from build123d import *

# Parameters (mm, degrees)
SKETCH1_W           = 90
SKETCH1_H           = 90
BOSS_EXTRUDE1_DEPTH = 25
SKETCH2_W           = 50
SKETCH2_H           = 25
BOSS_EXTRUDE2_DEPTH = 90
CUT_EXTRUDE1_DEPTH  = 114
BOSS_EXTRUDE3_DEPTH = 90
CUT_EXTRUDE2_DEPTH  = 90
CUT_EXTRUDE3_DEPTH  = 7
SKETCH12_W          = 60
SKETCH12_H          = 3.762713397
CUT_EXTRUDE4_DEPTH  = 7
SKETCH13_W          = 60
SKETCH13_H          = 6.597800351
BOSS_EXTRUDE4_DEPTH = 4
SKETCH15_W          = 60
SKETCH15_H          = 4.875511562
BOSS_EXTRUDE5_DEPTH = 6
CUT_EXTRUDE5_DEPTH  = 105
CUT_EXTRUDE6_DEPTH  = 105
CUT_EXTRUDE7_DEPTH  = 105
CUT_EXTRUDE8_DEPTH  = 105
SKETCH20_R          = 5.002398859
BOSS_EXTRUDE6_DEPTH = 5
SKETCH21_R          = 5.013240391
BOSS_EXTRUDE7_DEPTH = 5
CUT_EXTRUDE9_DEPTH  = 110
CUT_EXTRUDE10_DEPTH = 110
BOSS_EXTRUDE8_DEPTH = 90


with BuildPart() as part:
    # Sketch1 → Boss-Extrude1 (new body)
    with BuildSketch(Plane(origin=(0, 0, 0), x_dir=(1, 0, 0), z_dir=(0, 1, 0))):
        with Locations((-396.44486692, -394.733840304)):
            Rectangle(SKETCH1_W, SKETCH1_H)
    extrude(amount=BOSS_EXTRUDE1_DEPTH)

    # Sketch2 → Boss-Extrude2 (add)
    with BuildSketch(Plane(origin=(-351.44486692, 0, 0), x_dir=(0, 0, -1), z_dir=(1, 0, 0))):
        with Locations((-324.733840304, 12.5)):
            Rectangle(SKETCH2_W, SKETCH2_H)
    extrude(amount=-BOSS_EXTRUDE2_DEPTH)

    # Sketch3 → Cut-Extrude1 (cut)
    with BuildSketch(Plane(origin=(-351.44486692, 0, 0), x_dir=(0, 0, -1), z_dir=(1, 0, 0))):
        Polygon((-439.733840304, 0), (-431.428630034, 25), (-426.683614644, 23.423665978), (-432.80411144, 5), (-422.80411144, 5), (-417.80411144, 5), (-409.869768155, 28.88363156), (-456.556935105, 33.347834294), align=None)
    extrude(amount=-CUT_EXTRUDE1_DEPTH, mode=Mode.SUBTRACT)

    # Sketch6 → Boss-Extrude3 (add)
    with BuildSketch(Plane(origin=(-351.44486692, 0, 0), x_dir=(0, 0, -1), z_dir=(1, 0, 0))):
        Polygon((-417.80411144, 5), (-402.036905068, 52.448869357), (-397.292018132, 50.872148719), (-412.958326169, 3.726916659), align=None)
    extrude(amount=-BOSS_EXTRUDE3_DEPTH)

    # Sketch8 → Cut-Extrude2 (cut)
    with BuildSketch(Plane.ZY.offset(441.44486692)):
        Polygon((402.036905068, 52.448869357), (417.80411144, 5), (422.667757436, 11.843524049), (408.096373886, 67.204399508), align=None)
    extrude(amount=-CUT_EXTRUDE2_DEPTH, mode=Mode.SUBTRACT)

    # Sketch11 → Cut-Extrude3 (cut)
    with BuildSketch(Plane(origin=(0, 131.563601718, 396.027305256), x_dir=(1, 0, 0), z_dir=(0, 0.31526680439845073, 0.9490030779952134))):
        Polygon((-396.44486692, -112.290048567), (-366.44486692, -112.290048567), (-366.44486692, -132.290048567), (-426.44486692, -132.290048567), (-426.44486692, -112.290048567), align=None)
    extrude(amount=-CUT_EXTRUDE3_DEPTH, mode=Mode.SUBTRACT)

    # Sketch12 → Cut-Extrude4 (cut)
    with BuildSketch(Plane(origin=(0, 131.563601718, 396.027305256), x_dir=(1, 0, 0), z_dir=(0, 0.31526680439845073, 0.9490030779952134))):
        with Locations((-396.44486692, -134.171405266)):
            Rectangle(SKETCH12_W, SKETCH12_H)
    extrude(amount=-CUT_EXTRUDE4_DEPTH, mode=Mode.SUBTRACT)

    # Sketch13 → Boss-Extrude4 (add)
    with BuildSketch(Plane(origin=(0, 5, 0), x_dir=(1, 0, 0), z_dir=(0, 1, 0))):
        with Locations((-396.44486692, -433.995536892)):
            Rectangle(SKETCH13_W, SKETCH13_H)
    extrude(amount=-BOSS_EXTRUDE4_DEPTH)

    # Sketch15 → Boss-Extrude5 (add)
    with BuildSketch(Plane(origin=(0, 131.563601718, 396.027305256), x_dir=(1, 0, 0), z_dir=(0, 0.31526680439845073, 0.9490030779952134))):
        with Locations((-396.44486692, -133.615006183)):
            Rectangle(SKETCH15_W, SKETCH15_H)
    extrude(amount=-BOSS_EXTRUDE5_DEPTH)

    # Sketch16 → Cut-Extrude5 (cut)
    with BuildSketch(Plane.ZY.offset(441.44486692)):
        Polygon((299.733840304, 25), (405.889304299, 25), (320.938870245, 45.924702762), (282.519842095, 35.688976285), (299.733840304, -6.375653077), (299.733840304, 0), (299.733840304, 13.612271354), align=None)
        Polygon((409.673433828, 13.612271354), (405.889304299, 25), (299.733840304, 25), (299.733840304, 13.612271354), align=None)
    extrude(amount=-CUT_EXTRUDE5_DEPTH, mode=Mode.SUBTRACT)

    # Sketch17 → Cut-Extrude6 (cut)
    with BuildSketch(Plane(origin=(-351.44486692, 0, 0), x_dir=(0, 0, -1), z_dir=(1, 0, 0))):
        Polygon((-354.703637066, 13.612271354), (-354.703637066, -9.141758862), (-285.710269568, -9.141758862), (-285.710269568, 26.661614512), (-354.703637066, 26.661614512), align=None)
    extrude(amount=-CUT_EXTRUDE6_DEPTH, mode=Mode.SUBTRACT)

    # Sketch18 → Cut-Extrude7 (cut)
    with BuildSketch(Plane(origin=(0, 125.526947543, 377.753141183), x_dir=(1, 0, 0), z_dir=(0, 0.3153441274409663, 0.9489773871323255))):
        Polygon((-441.44486692, -77.007186028), (-436.44486692, -77.007186028), (-441.44486692, -82.007186028), align=None)
    extrude(amount=-CUT_EXTRUDE7_DEPTH, mode=Mode.SUBTRACT)

    # Sketch19 → Cut-Extrude8 (cut)
    with BuildSketch(Plane(origin=(0, 125.526947543, 377.753141183), x_dir=(1, 0, 0), z_dir=(0, 0.3153441274409663, 0.9489773871323255))):
        Polygon((-351.44486692, -82.007186028), (-351.44486692, -77.007186028), (-356.44486692, -77.007186028), align=None)
    extrude(amount=-CUT_EXTRUDE8_DEPTH, mode=Mode.SUBTRACT)

    # Sketch20 → Boss-Extrude6 (add)
    with BuildSketch(Plane(origin=(0, 125.526947543, 377.753141183), x_dir=(1, 0, 0), z_dir=(0, 0.3153441274409663, 0.9489773871323255))):
        with Locations((-436.44486692, -82.007186028)):
            Circle(SKETCH20_R)
    extrude(amount=-BOSS_EXTRUDE6_DEPTH)

    # Sketch21 → Boss-Extrude7 (add)
    with BuildSketch(Plane(origin=(0, 125.526947543, 377.753141183), x_dir=(1, 0, 0), z_dir=(0, 0.3153441274409663, 0.9489773871323255))):
        with Locations((-356.44486692, -82.007186028)):
            Circle(SKETCH21_R)
    extrude(amount=-BOSS_EXTRUDE7_DEPTH)

    # Sketch22 → Cut-Extrude9 (cut)
    with BuildSketch(Plane.ZY.offset(441.44486692)):
        with BuildLine():
            Line((352.286663655, 0), (351.925563617, 18.995212977))
            Line((351.925563617, 18.995212977), (405.563075233, 20.014865007))
            Line((405.563075233, 20.014865007), (409.673433828, 13.612271354))
            add(Edge.make_bspline(
                [(409.673433828, 13.612271354), (391.693864934, -0.348112278), (371.968229932, 0.006592141), (352.286663655, 0)],
                knots=[0, 0, 0, 0, 1, 1, 1, 1], degree=3))
        make_face()
    extrude(amount=-CUT_EXTRUDE9_DEPTH, mode=Mode.SUBTRACT)

    # Sketch23 → Cut-Extrude10 (cut)
    with BuildSketch(Plane(origin=(-351.44486692, 0, 0), x_dir=(0, 0, -1), z_dir=(1, 0, 0))):
        Polygon((-432.207797356, 6.794999958), (-432.80411144, 5), (-433.434645049, 3.101993844), (-418.434799695, 3.102045226), (-417.80411144, 5), (-417.309872164, 6.487333538), align=None)
    extrude(amount=-CUT_EXTRUDE10_DEPTH, mode=Mode.SUBTRACT)

    # Sketch24 → Boss-Extrude8 (add)
    with BuildSketch(Plane(origin=(-351.44486692, 0, 0), x_dir=(0, 0, -1), z_dir=(1, 0, 0))):
        Polygon((-439.733840304, 0), (-440.364373913, -1.898006156), (-355.334170675, -1.898006156), (-354.703637066, 0), align=None)
    extrude(amount=-BOSS_EXTRUDE8_DEPTH)


solid = part.part
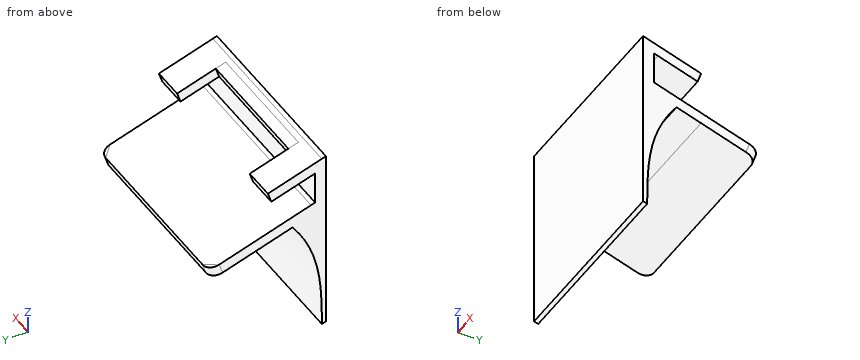
Geometry check sheet. Reference: the model listing, model coordinates, mm. Give positions to 0.01 mm unless a question says otherwise; leave off trailing zeros. Loops run counter-clockwise (first coordinate to the right, second up) from the corner with the lowest first, then second, coordinate; pieces in that order, holes last.
(1) Thickness scan on L1, parallel to X at y = 17, z = 434; L2, parallel to X at y = 1.5, z = 428; L3, parallel to Y at x = -361, z = 424.5. Record the ranges inside material, lowest first.
From the geometry:
L1: x = -441.44 to -426.44, -366.44 to -351.44
L2: x = -441.44 to -351.44
L3: y = -1.9 to 3.1
(2) Section check C-C on y = 42.5. Record the cut outline in (x, z).
From the geometry:
outline: (-441.44, 400.07) - (-351.44, 400.07) - (-351.44, 405.34) - (-441.44, 405.34) - close
(3) Section check A-A on y = 20.5. Record the cut outline in (x, z).
From the geometry:
outline: (-441.44, 407.38) - (-351.44, 407.38) - (-351.44, 412.65) - (-441.44, 412.65) - close; (-441.44, 427.65) - (-426.44, 427.65) - (-426.44, 432.92) - (-441.44, 432.92) - close; (-366.44, 427.65) - (-351.44, 427.65) - (-351.44, 432.92) - (-366.44, 432.92) - close
(4) Section check B-B on z = 429. Record the cut outline in (x, y), then the cut area to 3 significant figures.
From the geometry:
outline: (-441.44, -1.9) - (-351.44, -1.9) - (-351.44, 3.1) - (-441.44, 3.1) - close; (-441.44, 16.45) - (-426.44, 16.45) - (-426.44, 24.19) - (-441.44, 24.19) - close; (-366.44, 16.45) - (-351.44, 16.45) - (-351.44, 24.19) - (-366.44, 24.19) - close
area: 682 mm2
(5) Depth check by flat-ended pin: pin 1 Ø1 at (x, y) = (-404.5, 8.5) entering from -Z; pin 2 Ø4 at (x, y) = (-430.5, 38) entering from -Z; pin 3 Ø1 at (y, z) = (14, 408.5) entering from +X; pin 4 Ø0.6 at (y, z) = (0.5, 432.5) entering from -X. Enter the tip coordinate at first touch or a pass-through.
From the geometry:
pin 1: stops at z = 401.01
pin 2: stops at z = 400.9
pin 3: passes through
pin 4: stops at x = -441.44
